Verification items for the finished model (mm, model axes). Round coordinates to 2 decimals unless told otherwise and drop trailing zeros. Write each loop counter-clockwise with the first axis right and the second up, starting at its lowest first coordinate (ties: lowest second). Pieces come first, ordered by that corner, then holes. Notation, with made-up numbers: M -11.75,9 L 13.25,9 A22 cw 13.25,42 Z; hole C 27.25,38 d9. An arc over 180 degrees is marked long. One line per item, written item: value. Start each with the question number.
Item 1: Section check C-C, the plane x = 70. Record the cut outline in (y, z).
Item 2: Draft check along X on faces 1 (the face through (147, 0, -108)), 2 (the face through (21.713, 2.332, -46.672)), 3 (the face through (148.4, 2.3, -6.7)). Enter one of: +X half, -X half, draft (parallel to the pull), parting line (faces both ways), or undercut.
Item 3: Gauge pin test, flat ends, axial feed: pin 1 (1.9 mm diameter, centred on x = 162.69, z = -62.1, fed in from +Y); pin 2 (2 mm diameter, centred on x = 154.5, z = -57, fed in from -Y); pin 3 (1 mm diameter, centred on x = 171.5, y = 0.5, fed in from +Z). Record the tip position at first contact, or that the pin passes through.
Item 4: Section check B-B, the plane y = 1.6. State how many separate pieces and enclosed holes the cut face has, then the cut area to 3 significant figures.
Item 5: Thickness scan on probe 1 along Z at (x, y) = (149, 2.65); probe 2 along X at (y, z) = (2.1, -85.81); probe 3 along X at (y, z) = (2.4, -56). Record the ranges inside material, lowest first. Write a range as from..to.
Item 6: Section check A-A, the plane z = -113.5. Record the cut outline in (x, y), then the cut area to 3 significant figures.
Item 7: Section check D-D, the plane x = 188.5. Record the cut outline in (y, z).
from build123d import *

# Parameters (mm, degrees)
ESQUISSE2_W                = 298
ESQUISSE2_H                = 145
BOSS_EXTRU_1_DEPTH         = 4.6
CREUX_STOCKAGE_VERRE_DEPTH = 46.6
ESQUISSE6_R                = 10.25
TROU_BILLE_DEPTH           = 5.6
ESQUISSE7_R                = 1.6
ENL_V_MAT_EXTRU_3_DEPTH    = 5.6
ENL_V_MAT_EXTRU_7_DEPTH    = 29
ESQUISSE17_R               = 1.6
ENL_V_MAT_EXTRU_14_DEPTH   = 4.6
BOSS_EXTRU_5_DEPTH         = 4.6
ENL_V_MAT_EXTRU_15_DEPTH   = 4.6
ENL_V_MAT_EXTRU_16_DEPTH   = 4.6
ESQUISSE12_R               = 2.25
ENL_V_MAT_EXTRU_17_DEPTH   = 10


with BuildPart() as part:
    # Esquisse2 → Boss.-Extru.1 (new body)
    with BuildSketch(Plane(origin=(0, 0, 0), x_dir=(1, 0, 0), z_dir=(0, 1, 0))):
        with Locations((149, 72.5)):
            Rectangle(ESQUISSE2_W, ESQUISSE2_H)
    extrude(amount=BOSS_EXTRU_1_DEPTH)

    # Esquisse3 → creux_stockage_verre (cut)
    with BuildSketch(Plane(origin=(0, 4.6, 0), x_dir=(1, 0, 0), z_dir=(0, 1, 0))):
        with BuildLine():
            Line((46, 83), (42, 0))
            Line((42, 0), (124, 0))
            Line((124, 0), (120, 83))
            ThreePointArc((120, 83), (83, 120), (46, 83))
        make_face()
        with BuildLine():
            Line((174, 0), (256, 0))
            Line((256, 0), (252, 83))
            ThreePointArc((252, 83), (215, 120), (178, 83))
            Line((178, 83), (174, 0))
        make_face()
    extrude(amount=-CREUX_STOCKAGE_VERRE_DEPTH, mode=Mode.SUBTRACT)

    # Esquisse6 → trou_bille (cut, through all)
    with BuildSketch(Plane(origin=(0, 4.6, 0), x_dir=(1, 0, 0), z_dir=(0, 1, 0))):
        with Locations((149, 70)):
            Circle(ESQUISSE6_R)
    extrude(amount=-TROU_BILLE_DEPTH, mode=Mode.SUBTRACT)

    # Esquisse7 → Enlèv. mat.-Extru.3 (cut, through all)
    with BuildSketch(Plane(origin=(0, 4.6, 0), x_dir=(1, 0, 0), z_dir=(0, 1, 0))):
        with Locations((32.5, 134)):
            Circle(ESQUISSE7_R)
        with Locations((80.5, 134)):
            Circle(ESQUISSE7_R)
        with Locations((128.5, 134)):
            Circle(ESQUISSE7_R)
        with Locations((217.5, 134)):
            Circle(ESQUISSE7_R)
        with Locations((169.5, 134)):
            Circle(ESQUISSE7_R)
        with Locations((265.5, 134)):
            Circle(ESQUISSE7_R)
    extrude(amount=-ENL_V_MAT_EXTRU_3_DEPTH, mode=Mode.SUBTRACT)

    # Esquisse9 → Enlèv. mat.-Extru.7 (cut)
    with BuildSketch(Plane(origin=(0, 4.6, 0), x_dir=(1, 0, 0), z_dir=(0, 1, 0))):
        with BuildLine():
            Line((123.101131567, 18.651519988), (120.058616356, -9.942070174))
            Line((120.058616356, -9.942070174), (178.789756957, -9.942070174))
            Line((178.789756957, -9.942070174), (174.898868433, 18.651519988))
            ThreePointArc((174.898868433, 18.651519988), (149, 12.489846239), (123.101131567, 18.651519988))
        make_face()
    extrude(amount=-ENL_V_MAT_EXTRU_7_DEPTH, mode=Mode.SUBTRACT)

    # Esquisse17 → Enlèv. mat.-Extru.14 (cut)
    with BuildSketch(Plane(origin=(0, 4.6, 0), x_dir=(1, 0, 0), z_dir=(0, 1, 0))):
        with Locations((149, 85.81)):
            Circle(ESQUISSE17_R)
        with Locations((135.308138366, 62.095)):
            Circle(ESQUISSE17_R)
        with Locations((162.691861634, 62.095)):
            Circle(ESQUISSE17_R)
    extrude(amount=-ENL_V_MAT_EXTRU_14_DEPTH, mode=Mode.SUBTRACT)

    # Esquisse15 → Boss.-Extru.5 (add)
    with BuildSketch(Plane(origin=(0, 4.6, 0), x_dir=(1, 0, 0), z_dir=(0, 1, 0))):
        with BuildLine():
            ThreePointArc((175.493975904, 31), (149, 6), (122.506024096, 31))
            ThreePointArc((122.506024096, 31), (149, 25.792591017), (175.493975904, 31))
        make_face()
    extrude(amount=-BOSS_EXTRU_5_DEPTH)

    # Esquisse18 → Enlèv. mat.-Extru.15 (cut)
    with BuildSketch(Plane(origin=(0, 4.6, 0), x_dir=(1, 0, 0), z_dir=(0, 1, 0))):
        with BuildLine():
            Line((175.493975904, 31), (178.847567105, -7.009778322))
            Line((178.847567105, -7.009778322), (115.973210985, -7.009778322))
            Line((115.973210985, -7.009778322), (122.506024096, 31))
            ThreePointArc((122.506024096, 31), (149, 6.694262171), (175.493975904, 31))
        make_face()
    extrude(amount=-ENL_V_MAT_EXTRU_15_DEPTH, mode=Mode.SUBTRACT)

    # Esquisse14 → Enlèv. mat.-Extru.16 (cut)
    with BuildSketch(Plane(origin=(0, 4.6, 0), x_dir=(1, 0, 0), z_dir=(0, 1, 0))):
        with BuildLine():
            Line((0, 71.707789669), (-22.158835411, -9.528975932))
            Line((-22.158835411, -9.528975932), (50.380974376, -9.528975932))
            Line((50.380974376, -9.528975932), (45.101419153, 64.354447432))
            ThreePointArc((45.101419153, 64.354447432), (19.112822484, 46.944980874), (0, 71.707789669))
        make_face()
        with BuildLine():
            Line((252.898580847, 64.354447432), (243.707235712, -12.373693019))
            Line((243.707235712, -12.373693019), (332.150206643, -12.373693019))
            Line((332.150206643, -12.373693019), (298, 71.707789669))
            ThreePointArc((298, 71.707789669), (279.381330699, 43.914112857), (252.898580847, 64.354447432))
        make_face()
    extrude(amount=-ENL_V_MAT_EXTRU_16_DEPTH, mode=Mode.SUBTRACT)

    # Esquisse12 → Enlèv. mat.-Extru.17 (cut)
    with BuildSketch(Plane(origin=(0, 4.6, 0), x_dir=(1, 0, 0), z_dir=(0, 1, 0))):
        with Locations((27, 64)):
            Circle(ESQUISSE12_R)
        with Locations((149, 134)):
            Circle(ESQUISSE12_R)
        with Locations((271, 64)):
            Circle(ESQUISSE12_R)
    extrude(amount=-ENL_V_MAT_EXTRU_17_DEPTH, mode=Mode.SUBTRACT)


solid = part.part
Response values:
1. outline: M 0,-145 L 4.6,-145 L 4.6,-117.64 L 0,-117.64 Z
2. face 1: draft
2. face 2: undercut
2. face 3: parting line
3. pin 1: passes through
3. pin 2: stops at y = 0
3. pin 3: stops at z = -18.35
4. separate pieces: 1
4. enclosed holes: 13
4. area: 20,600 mm2
5. probe 1: z = -145..-136.25, -131.75..-87.41, -84.21..-80.25, -59.75..-6.69
5. probe 2: x = 0..46.11, 119.89..147.4, 150.6..178.11, 251.89..298
5. probe 3: x = 4.33..41.26, 121.3..176.7, 255.35..296.04
6. outline: M 0,0 L 62.05,0 L 62.05,4.6 L 0,4.6 Z; M 103.95,0 L 194.05,0 L 194.05,4.6 L 103.95,4.6 Z; M 235.95,0 L 298,0 L 298,4.6 L 235.95,4.6 Z
6. area: 985 mm2
7. outline: M 0,-145 L 4.6,-145 L 4.6,-108.82 L 0,-108.82 Z
